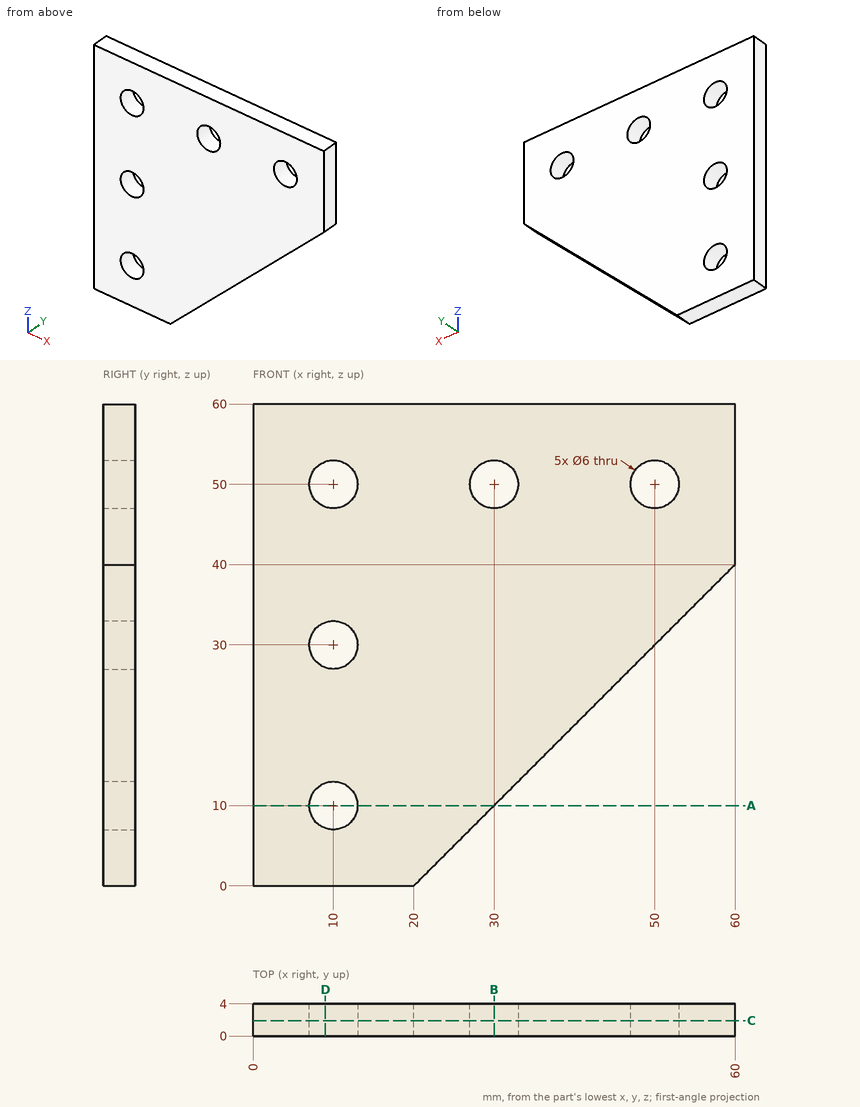
Drawing for the job (mm, zero at the part's lowest x, y, z). Coordinates: 2 decimals unless noted, no trailing zeros. Loops run counter-clockwise (first coordinate to the right, second up) from the corner with the lowest first, then second, coordinate; pieces in that order, holes last. Notation, with made-up numbers: (-13, 9) - (40, 9) arc R16 cw to (40, 30) - close; hole circle Ø1 at (-29.5, -5.5). An arc over 180 degrees is marked (long way). Return JSON: item names as keys, results as strings.
1. Drop flat-ended pins along their axis: pin 1 (3.5 mm diameter, centred on x = 50, z = 50, fed in from +Y); pin 2 (8 mm diameter, centred on x = 10, z = 30, fed in from -Y); pin 3 (1.5 mm diameter, centred on y = 3, z = 19, fed in from +X). Give the stop position or say it passes through.
Result:
{"pin 1": "passes through", "pin 2": "stops at y = 0", "pin 3": "stops at x = 39.75"}
2. Band-saw the part on B-B (x = 30). Give the cut face in (y, z), and give its area (3 significant figures).
Result:
{"outline": "(0, 10) - (4, 10) - (4, 47) - (0, 47) - close; (0, 53) - (4, 53) - (4, 60) - (0, 60) - close", "area": "176 mm2"}
3. Band-saw the part on A-A (z = 10). Give the cut face in (x, y).
Result:
{"outline": "(0, 0) - (7, 0) - (7, 4) - (0, 4) - close; (13, 0) - (30, 0) - (30, 4) - (13, 4) - close"}
4. Band-saw the part on C-C (y = 1.9). Give the cut face in (x, z), and give its area (3 significant figures).
Result:
{"outline": "(0, 0) - (20, 0) - (60, 40) - (60, 60) - (0, 60) - close; hole circle Ø6 at (10, 10); hole circle Ø6 at (10, 30); hole circle Ø6 at (10, 50); hole circle Ø6 at (30, 50); hole circle Ø6 at (50, 50)", "area": "2,660 mm2"}
5. Probe L1, parallel to X at y = 2.25, z = 50; L2, parallel to Z at x = 9, y = 3.4. List the from-to ranges inside material, lowest first. Write a range as from..to.
Result:
{"L1": "x = 0..7, 13..27, 33..47, 53..60", "L2": "z = 0..7.17, 12.83..27.17, 32.83..47.17, 52.83..60"}
6. Band-saw the part on D-D (x = 9). Give the cut face in (y, z).
Result:
{"outline": "(0, 0) - (4, 0) - (4, 7.17) - (0, 7.17) - close; (0, 12.83) - (4, 12.83) - (4, 27.17) - (0, 27.17) - close; (0, 32.83) - (4, 32.83) - (4, 47.17) - (0, 47.17) - close; (0, 52.83) - (4, 52.83) - (4, 60) - (0, 60) - close"}
